```python
from build123d import *

# Parameters (mm, degrees)
F1_DEPTH = 25


with BuildPart() as f1:
    # F0 (on Top) → F1 (new body)
    with BuildSketch(Plane.XY):
        with BuildLine():
            ThreePointArc((-19.63329, 30.391514), (-9.816645, 32.135515), (0, 30.391514))
            Line((0, 30.391514), (0, -30.391514))
            ThreePointArc((0, -30.391514), (-9.816645, -32.135515), (-19.63329, -30.391514))
            ThreePointArc((-19.63329, -30.391514), (-22.525582, -31.645534), (-21.415574, -34.596093))
            ThreePointArc((-21.415574, -34.596093), (-8.951554, -37.435962), (3.5, -34.541927))
            Line((3.5, -34.541927), (3.5, 34.541927))
            ThreePointArc((3.5, 34.541927), (-8.951554, 37.435962), (-21.415574, 34.596093))
            ThreePointArc((-21.415574, 34.596093), (-22.525582, 31.645534), (-19.63329, 30.391514))
        make_face()
    extrude(amount=F1_DEPTH)


solid = f1.part
```
Input: part model. Units: mm. Frame: model coordinates. A direction names the side the tool comes from. Give positions to 0.01 mm unless a question says otherwise; leave off trailing zeros. Order: outer loops, then holes, each group sorted by start corner. A loop starts at its lowest first (then second) coordinate and runs counter-clockwise, first axis right, second up.
1. Section A-A on x = -13.5. Return the cut outline in (y, z).
Derived:
outline: (-37.08, 0) - (-31.9, 0) - (-31.9, 25) - (-37.08, 25) - close; (31.9, 0) - (37.08, 0) - (37.08, 25) - (31.9, 25) - close
2. Section D-D on x = -10.5. Return the cut outline in (y, z).
Derived:
outline: (-37.4, 0) - (-32.13, 0) - (-32.13, 25) - (-37.4, 25) - close; (32.13, 0) - (37.4, 0) - (37.4, 25) - (32.13, 25) - close
3. Mould query, pull axis Y, two halves, no side actions, for faces 3 (the cylindrical face through (-8.771, 37.435, 12.325)), 4 (the flat face through (0, 0, 12)), 5 (the flat face through (1, -3, 0)), 6 (the cylindrical face through (-9.132, -37.436, 12.325)). Classes: released by +Y, released by -Y, zero draft, split by the parting line, or undercut.
Derived:
face 3: released by +Y
face 4: undercut
face 5: zero draft
face 6: released by -Y
4. Reachability of faces 1 (the cylindrical face through (-9.676, -32.135, 12.325)), 2 (the flat face through (3.5, 0, 12)) from +Z, -Z, +X, -X, +Y, -Y: full face, straight path, thin tool, end or side. Return the list, or none.
Derived:
face 1: +Z, -Z
face 2: +Z, -Z, +X, +Y, -Y
5. Section B-B on z = 7. Return the cut outline in (x, y), and give its area (3 significant figures).
Derived:
outline: (-21.42, -34.6) arc R28.5 ccw to (3.5, -34.54) - (3.5, 34.54) arc R28.5 ccw to (-21.42, 34.6) arc R2.29 ccw to (-19.63, 30.39) arc R28.5 cw to (0, 30.39) - (0, -30.39) arc R28.5 cw to (-19.63, -30.39) arc R2.29 ccw to start
area: 479 mm2
6. Material intervals for L1, parallel to Y at x = -9.25, z = 12; L2, parallel to X at y = 18, z = 23.5; L3, parallel to Y at x = -15.25, z = 16.75, sorted ascending.
Derived:
L1: y = -37.44 to -32.13, 32.13 to 37.44
L2: x = 0 to 3.5
L3: y = -36.75 to -31.61, 31.61 to 36.75
7. Section C-C on y = -7. Return the cut outline in (x, z), and give its area (3 significant figures).
Derived:
outline: (0, 0) - (3.5, 0) - (3.5, 25) - (0, 25) - close
area: 87.5 mm2
8. Pin query (flat end, axial travel): pin 1 (8 mm diameter, centred on y = 18, z = 21.5, fed in from -X); pin 2 (2 mm diameter, centred on x = -16, z = 19, fed in from -Y); pin 3 (10 mm diameter, centred on x = -3.5, z = 6.5, fed in from -Y). Return the tip coordinate at first contact, or that it passes through.
Derived:
pin 1: stops at x = 0
pin 2: stops at y = -36.8
pin 3: stops at y = -37.43
